from build123d import *

# Parameters (mm, degrees)
F7_T      = -0.5
F12_DEPTH = 1
F13_DEPTH = 1
F14_DEPTH = 1
F15_DEPTH = 1
F21_DEPTH = 1
F22_DEPTH = 1
F23_DEPTH = 1
F24_DEPTH = 1
F25_DEPTH = 1


with BuildPart() as f3:
    # F0 (on Top) → F3 section 0
    with BuildSketch(Plane.XY):
        Polygon((-6.4983939247, -8.94427191), (6.4983939247, -8.94427191), (10.5146222424, 3.416407865), (0, 11.05572809), (-10.5146222424, 3.416407865), align=None)
    # F2 (on offset) → F3 section 1
    with BuildSketch(Plane.XY.offset(22)):
        Polygon((-0.0324919696, -0.0447213595), (0.0324919696, -0.0447213595), (0.0525731112, 0.0170820393), (0, 0.0552786405), (-0.0525731112, 0.0170820393), align=None)
    loft()

    # F3_face (on face) → F6 section 0
    with BuildSketch(Plane(origin=(0, 0, 0), x_dir=(1, 0, 0), z_dir=(0, 0, -1))):
        Polygon((6.4983939247, 8.94427191), (-6.4983939247, 8.94427191), (-10.5146222424, -3.416407865), (0, -11.05572809), (10.5146222424, -3.416407865), align=None)
    # F5 (on offset) → F6 section 1
    with BuildSketch(Plane.XY.offset(-12)):
        Polygon((-1.9495181774, -2.683281573), (1.9495181774, -2.683281573), (3.1543866727, 1.0249223595), (0, 3.316718427), (-3.1543866727, 1.0249223595), align=None)
    loft()

    # F7
    f7_openings = [f3.faces().sort_by_distance(p)[0] for p in [
        (-3.504961, 4.824165, 7.369818),
    ]]
    offset(amount=F7_T, openings=f7_openings)

    # F11 (on face) → F12 (cut)
    with BuildSketch(Plane(origin=(4.5179857008, 6.2184738355, 3.1093639582), x_dir=(-0.8385071819, 0.4873609368, 0.2436904249), z_dir=(0.5448905449, 0.7499774946, 0.375004069))):
        Polygon((4.8481299984, 17.7941495307), (-6.3276584478, -1.1927079159), (4.8481299984, -4.237623051), align=None)
    extrude(amount=-F12_DEPTH, mode=Mode.SUBTRACT)

    # F10 (on face) → F13 (cut)
    with BuildSketch(Plane(origin=(7.3102544246, -2.375245647, 3.1093639582), x_dir=(0.2636108968, 0.9580904348, 0.1121249924), z_dir=(0.8816514217, -0.2864659121, 0.375004069))):
        Polygon((2.2306848501, 18.3073801267), (-6.0894386648, -2.0929764337), (5.4086892422, -3.4939797203), align=None)
    extrude(amount=-F13_DEPTH, mode=Mode.SUBTRACT)

    # F8 (on face) → F14 (cut)
    with BuildSketch(Plane(origin=(-7.3102544246, -2.375245647, 3.1093639582), x_dir=(0.2636108968, -0.9580904348, -0.1121249924), z_dir=(-0.8816514217, -0.2864659121, 0.375004069))):
        Polygon((-2.2311449625, 18.3111563002), (-5.4098675893, -3.4951306933), (6.0908589153, -2.0938107774), align=None)
    extrude(amount=-F14_DEPTH, mode=Mode.SUBTRACT)

    # F9 (on face) → F15 (cut)
    with BuildSketch(Plane(origin=(0, -7.686456377, 3.1093639582), x_dir=(1, 0, 0), z_dir=(0, -0.9270231649, 0.375004069))):
        Polygon((0, 18.4427796713), (-5.7915834531, -2.8141383603), (5.7915834531, -2.8141383603), align=None)
    extrude(amount=-F15_DEPTH, mode=Mode.SUBTRACT)

    # F20 (on face) → F21 (cut)
    with BuildSketch(Plane(origin=(6.6863382316, -2.1725229871, -3.6681222707), x_dir=(0.2401975954, 0.9617386219, -0.1317722973), z_dir=(0.843188815, -0.2739686536, -0.4625730203))):
        Polygon((2.8605048602, -8.5273181822), (5.1487184249, 4.4116316912), (-6.2180731217, 2.7032133195), (-0.2274522358, -8.9914353091), align=None)
    extrude(amount=-F21_DEPTH, mode=Mode.SUBTRACT)

    # F16 (on face) → F22 (cut)
    with BuildSketch(Plane(origin=(4.1323842874, 5.6877390216, -3.6681222707), x_dir=(-0.8534838174, 0.4379434765, -0.2824373997), z_dir=(0.5211193466, 0.7172592471, -0.4625730203))):
        Polygon((4.3017839952, -7.8988795342), (4.3017839952, 5.240844403), (-6.5938117294, 1.5790637972), (1.3418342156, -8.893656412), align=None)
    extrude(amount=-F22_DEPTH, mode=Mode.SUBTRACT)

    # F19 (on face) → F23 (cut)
    with BuildSketch(Plane(origin=(0, -7.030432069, -3.6681222707), x_dir=(1, 0, 0), z_dir=(0, -0.8865811868, -0.4625730203))):
        Polygon((1.5613202534, -8.8577605806), (5.7472307114, 3.597378872), (-5.7472307114, 3.597378872), (-1.5613202534, -8.8577605806), align=None)
    extrude(amount=-F23_DEPTH, mode=Mode.SUBTRACT)

    # F18 (on face) → F24 (cut)
    with BuildSketch(Plane(origin=(-6.6863382316, -2.1725229871, -3.6681222707), x_dir=(0.2401975954, -0.9617386219, 0.1317722973), z_dir=(-0.843188815, -0.2739686536, -0.4625730203))):
        Polygon((0.2274522358, -8.9914353091), (6.2180731217, 2.7032133195), (-5.1487184249, 4.4116316912), (-2.8605048602, -8.5273181822), align=None)
    extrude(amount=-F24_DEPTH, mode=Mode.SUBTRACT)

    # F17 (on face) → F25 (cut)
    with BuildSketch(Plane(origin=(-4.1323842874, 5.6877390216, -3.6681222707), x_dir=(-0.8534838174, -0.4379434765, 0.2824373997), z_dir=(-0.5211193466, 0.7172592471, -0.4625730203))):
        Polygon((-1.3418342156, -8.893656412), (6.5938117294, 1.5790637972), (-4.3017839952, 5.240844403), (-4.3017839952, -7.8988795342), align=None)
    extrude(amount=-F25_DEPTH, mode=Mode.SUBTRACT)


solid = f3.part
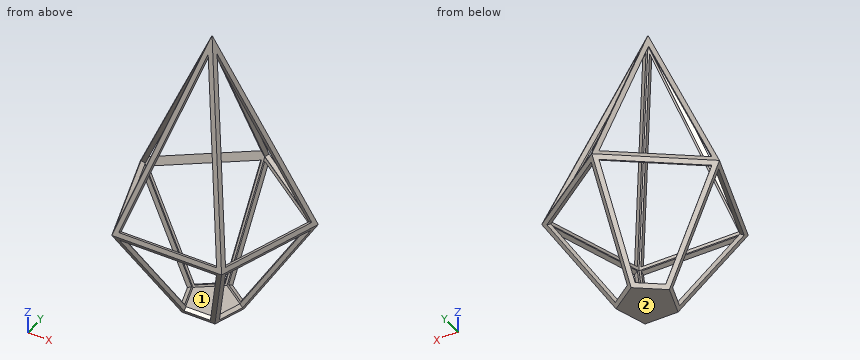
Part model, mm, in its own coordinate system. Face numbers are marked on the shaded views. Round coordinates to 2 decimals unless told otherwise and drop trailing zeros. Return JSON: item names as keys, results as strings. Group by question number.
(1) Saw through at A-A on x = -7.5. Count the separate pieces of the cut face and the enclosed holes in it, then the cut area to 3 significant figures.
(2) Drill centre lines: probe 1 along Z at (x, y) = (-9, -1); probe 2 along Y at (x, z) = (2, 15). Where is each one in solid material? Low to high.
(3) Two-plate mould, pull along Y, no slides. Class the marked faces 1 and 2: +Y half, -Y half, draft (parallel to the pull), parting line (faces both ways), or undercut.
(4) Pin check, flat tips, straight feed: pin 1 Ø6 at (x, y) = (0.5, 7.5) entering from -Z; pin 2 Ø1.6 at (x, y) = (1.5, 1) entering from +Z; pin 3 Ø1.5 at (x, y) = (-4.5, 7.5) entering from -Z; pin 4 Ø1 at (x, y) = (-4, -3) entering from -Z. Stop position of each tip, or through.
Returned:
{
 "1": {"separate pieces": "4", "enclosed holes": "0", "area": "3.35 mm²"},
 "2": {"probe 1": "-0.15 to 0.19", "probe 2": "-2.88 to -2.23"},
 "3": {"face 1": "undercut", "face 2": "draft"},
 "4": {"pin 1": "z = -10.1", "pin 2": "z = 19.91", "pin 3": "z = -0.48", "pin 4": "through"}
}
